Could you check a few things on this model? Use its own coordinates, in mm. A direction names the side the tool comes from. Give positions to 0.01 mm unless a question says otherwise; leave off trailing zeros. Loops run counter-clockwise (first coordinate to the right, second up) from the corner with the lowest first, then second, coordinate; pieces in that order, holes last. Notation, with made-up numbers: (53, -4) -> (78, -4) arc R19 ccw to (78, 19) -> close; hole circle Ø3 at (16.25, 19.5). An arc over 180 degrees is marked (long way). Write item = value, one per line. Start each with the question number.
1) I want a section at B-B (x = 1.25). List the corners of the cut face in (y, z) for me, and give its area (3 significant figures).
2) I want a section at D-D (x = 4.5). List the corners of the cut face in (y, z) for me, and give its area (3 significant figures).
3) I'm going to push flat-ended pins straight in: pin 1 Ø4 at (y, z) = (-2, 4) entering from +X; pin 2 Ø5.5 at (x, y) = (0, 0) entering from -Z; pin 3 Ø2 at (x, z) = (-2, 2.5) entering from -Y; pin 4 Ø3 at (x, y) = (0, 0) entering from +Z. Where does each tip first touch, or does it pass through?
4) I want a section at A-A (y = 0). List the corners of the cut face in (x, z) for me.
5) I want a section at C-C (z = 4). List the corners of the cut face in (x, y) for me, and give its area (3 significant figures).
6) If we mould it in two halves opening along Y, with no side actions, what happens to faces 3 (the face through (6, 0, 15)), 4 (the face through (3.042, 5.172, 14.958)), 5 (the face through (0, -2, 15))? For each: +Y half, -Y half, draft (parallel to the pull), parting line (faces both ways), or undercut.
7) On a 3-axis mill with a long thin cutter (end or side, diameter ignored), from which of +Z, -Z, +X, -X, +Y, -Y can I reach the whole of each face in a straight line? I mean faces 1 (the face through (1, -2, 18)), 2 (the face through (-3, 0, 6)). Say none if no direction works.
8) I need wall thicknesses on probe 1 along X at (y, z) = (0, 15.85); probe 2 along Y at (x, z) = (0, 2.75); probe 3 along Y at (x, z) = (2.75, 11.5). Which ranges of each line are inside material? Lowest first, please. Write a range as from..to.
Autodesk Fusion 360 part; units mm, degrees
sketch "Sketch1" plane through (0, 0, 0) normal (0, 0, 1) x (1, 0, 0) in component "Component"
  circle A0 centre (0, 0) radius 5.75
  circle A1 centre (0, 0) radius 3
  dimension "d1" = 11.5
  dimension "d2" = 6
extrude "Extrude1" add sketch "Sketch1" along normal blind 12 in component "Component"
sketch "Sketch2" plane through (0, 0, 12) normal (0, 0, 1) x (-1, 0, 0) in component "Component"
  circle A0 centre (0, 0) radius 3
  circle A1 centre (0, 0) radius 5.75
  circle A2 centre (0, 0) radius 2
  line L0 (-6, 3.4641) -> (-6, -3.4641)
  line L1 (-6, -3.4641) -> (0, -6.9282)
  line L2 (0, -6.9282) -> (6, -3.4641)
  line L3 (6, -3.4641) -> (6, 3.4641)
  line L4 (6, 3.4641) -> (0, 6.9282)
  line L5 (0, 6.9282) -> (-6, 3.4641)
  dimension "d5" = 4
  dimension "d6" = 6
extrude "Extrude2" add sketch "Sketch2" along normal blind 6 contours A0 | A1 | L0 L1 L2 L3 L4 L5 in component "Component"
component "Component" placed x (1, 0, 0) y (0, 1, 0) z (0, 0, 1) at (0, 0, 0)
Answer list:
q1.outline = (-6.21, 12) -> (-5.61, 12) -> (-5.61, 0) -> (-2.73, 0) -> (-2.73, 12) -> (-1.56, 12) -> (-1.56, 18) -> (-6.21, 18) -> close; (1.56, 12) -> (2.73, 12) -> (2.73, 0) -> (5.61, 0) -> (5.61, 12) -> (6.21, 12) -> (6.21, 18) -> (1.56, 18) -> close
q1.area = 125 mm^2
q2.outline = (-4.33, 12) -> (-3.58, 12) -> (-3.58, 0) -> (3.58, 0) -> (3.58, 12) -> (4.33, 12) -> (4.33, 18) -> (-4.33, 18) -> close
q2.area = 138 mm^2
q3.pin_1 = 5.75
q3.pin_2 = 12
q3.pin_3 = -5.66
q3.pin_4 = through
q4.outline = (-6, 12) -> (-5.75, 12) -> (-5.75, 0) -> (-3, 0) -> (-3, 12) -> (-2, 12) -> (-2, 18) -> (-6, 18) -> close; (2, 12) -> (3, 12) -> (3, 0) -> (5.75, 0) -> (5.75, 12) -> (6, 12) -> (6, 18) -> (2, 18) -> close
q5.outline = circle Ø11.5 at (0, 0); hole circle Ø6 at (0, 0)
q5.area = 75.6 mm^2
q6.face_3 = draft
q6.face_4 = +Y half
q6.face_5 = undercut
q7.face_1 = +Z, +X, -X, +Y, -Y
q7.face_2 = -Z
q8.probe_1 = -6..-2, 2..6
q8.probe_2 = -5.75..-3, 3..5.75
q8.probe_3 = -5.05..-1.2, 1.2..5.05
